Geometry: see drawing. Coordinates: mm, zero at the bounding-box minimum. Give positions to 0.01 mm unless a question says otherwise; leave off trailing zeros. Write each loop counter-clockwise with the first axis right and the second up, starting at its lowest first coordinate (ties: lowest second). Pieces come first, ordered by that corner, then holes.
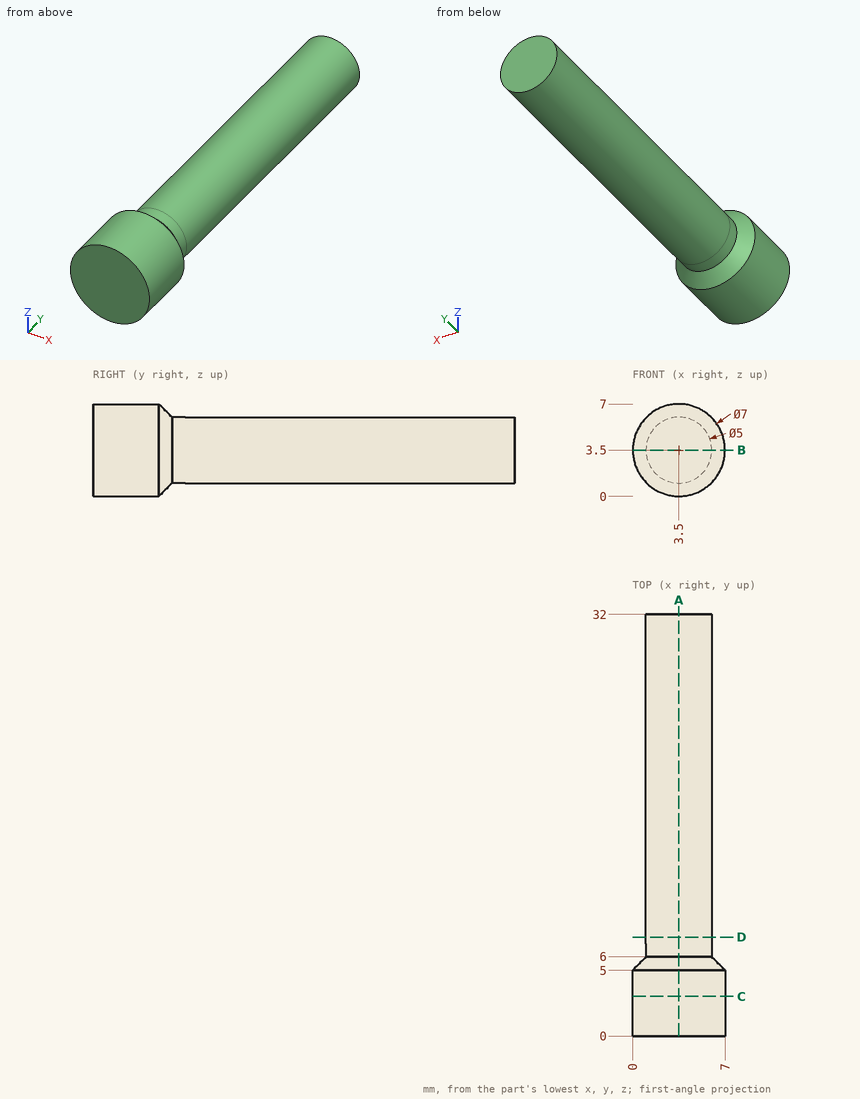
1. Line query: probe 1 along X at (y, z) = (8, 2.25); probe 2 along Z at (x, y) = (4.5, 22); probe 3 along X at (y, z) = (20, 1.5). Output: solid intervals per line, ascending.
2. Section query A-A (x = 3.5). Return loops of the section in (y, z).
3. Section query D-D (y = 7.5). Return loops of the section in (x, z).
4. Pin query (flat end, axial travel): P1, Ø1, axis at x = 3, z = 6, coming from the -Y side. Return the tip coordinate at first contact, or that it passes through.
5. Section query B-B (z = 3.5). Return loops of the section in (x, y).
6. Section query C-C (y = 3). Return loops of the section in (x, z).
The answers:
1. probe 1: x = 1.33 to 5.67
1. probe 2: z = 1.21 to 5.79
1. probe 3: x = 2 to 5
2. outline: (0, 0) - (5, 0) - (6, 1) - (32, 1) - (32, 6) - (6, 6) - (5, 7) - (0, 7) - close
3. outline: circle Ø5 at (3.5, 3.5)
4. P1: stops at y = 0
5. outline: (0, 0) - (7, 0) - (7, 5) - (6, 6) - (6, 32) - (1, 32) - (1, 6) - (0, 5) - close
6. outline: circle Ø7 at (3.5, 3.5)
